Check sheet for the modelled part. Datum: model origin and axes. Units: mm. A direction names the side the tool comes from. Coordinates: 2 decimals unless noted, no trailing zeros. Write each loop counter-clockwise with the first axis right and the second up, starting at its lowest first coordinate (ties: lowest second). Pieces come first, ordered by that corner, then holes. Notation, with made-up numbers: (18, 85) - (22, 85) arc R21 ccw to (22, 97) - close; hole circle Ø3 at (-33.5, 39). An arc over 180 degrees is marked (long way). Answer as CSV lines item,"result". Start each with the question number.
from build123d import *
from build123d.topology import SkipClean

# Parameters (mm, degrees)
SKETCH1_R           = 21
SKETCH1_R_2         = 2.2
BOSS_EXTRUDE1_DEPTH = 7
SKETCH3_R           = 11.25
SKETCH3_R_2         = 2
BOSS_EXTRUDE2_DEPTH = 14
CUT_EXTRUDE1_START  = -1.5
SKETCH4_R           = 11.25
SKETCH4_R_2         = 9.9
CUT_EXTRUDE1_DEPTH  = 1.5
SKETCH5_R           = 2.2
CUT_EXTRUDE2_DEPTH  = 133.951156445
CUT_EXTRUDE3_DEPTH  = 6.5
CUT_EXTRUDE4_START  = -10
SKETCH7_R           = 2
CUT_EXTRUDE4_DEPTH  = 10
SKETCH8_R           = 2.2
CUT_EXTRUDE5_DEPTH  = 133.951156445
SKETCH9_R           = 4.15
CUT_EXTRUDE6_DEPTH  = 3
BOSS_EXTRUDE3_START = 17.5
SKETCH10_R          = 21
SKETCH10_R_2        = 2.2
BOSS_EXTRUDE3_DEPTH = 17.5
CUT_EXTRUDE7_DEPTH  = 17.5


with BuildPart() as part:
    # Sketch1 → Boss-Extrude1 (new body)
    with BuildSketch(Plane(origin=(0, 0, 0), x_dir=(1, 0, 0), z_dir=(0, 1, 0))):
        with BuildLine():
            Line((-112.6, -35.6), (-112.6, 35.6))
            Line((-112.6, 35.6), (-20.090163155, 64.440944627))
            ThreePointArc((-20.090163155, 64.440944627), (67.5, 0), (-20.090163155, -64.440944627))
            Line((-20.090163155, -64.440944627), (-112.6, -35.6))
        make_face()
        with Locations(Location((-77, 0, 0), (0, 0, 270))):
            Circle(SKETCH1_R, mode=Mode.SUBTRACT)
        with Locations(Location((-100.6, 23.6, 0), (0, 0, 270))):
            Circle(SKETCH1_R_2, mode=Mode.SUBTRACT)
        with Locations(Location((-100.6, -23.6, 0), (0, 0, 270))):
            Circle(SKETCH1_R_2, mode=Mode.SUBTRACT)
        with Locations(Location((-53.4, -23.6, 0), (0, 0, 270))):
            Circle(SKETCH1_R_2, mode=Mode.SUBTRACT)
        with Locations(Location((-53.4, 23.6, 0), (0, 0, 270))):
            Circle(SKETCH1_R_2, mode=Mode.SUBTRACT)
    extrude(amount=BOSS_EXTRUDE1_DEPTH)

    # Sketch3 → Boss-Extrude2 (add)
    with BuildSketch(Plane.XZ):
        with Locations(Location((0, 0, 0), (0, 0, 90))):
            Circle(SKETCH3_R)
        with Locations(Location((0, 0, 0), (0, 0, 270))):
            Circle(SKETCH3_R_2, mode=Mode.SUBTRACT)
    extrude(amount=BOSS_EXTRUDE2_DEPTH)

    # Sketch4 → Cut-Extrude1 (cut)
    with BuildSketch(Plane.XZ.offset(14).offset(CUT_EXTRUDE1_START)):
        with Locations(Location((0, 0, 0), (0, 0, 90))):
            Circle(SKETCH4_R)
        with Locations(Location((0, 0, 0), (0, 0, 270))):
            Circle(SKETCH4_R_2, mode=Mode.SUBTRACT)
    extrude(amount=CUT_EXTRUDE1_DEPTH, mode=Mode.SUBTRACT)

    # Sketch5 → Cut-Extrude2 (cut, through all)
    with BuildSketch(Plane.XZ.offset(14)):
        with Locations(Location((-7.6, 0, 0), (0, 0, 270))):
            Circle(SKETCH5_R)
        with Locations(Location((3.8, 6.581793069, 0), (0, 0, 270))):
            Circle(SKETCH5_R)
        with Locations(Location((3.8, -6.581793069, 0), (0, 0, 270))):
            Circle(SKETCH5_R)
    extrude(amount=-CUT_EXTRUDE2_DEPTH, mode=Mode.SUBTRACT)

    # Sketch6 → Cut-Extrude3 (cut)
    with BuildSketch(Plane(origin=(0, 7, 0), x_dir=(1, 0, 0), z_dir=(0, 1, 0))):
        Polygon((3.8, 2.33826859), (7.475, 4.460030829), (7.475, 8.703555308), (3.8, 10.825317547), (0.125, 8.703555308), (0.125, 4.460030829), align=None)
        Polygon((-7.6, -4.243524479), (-3.925, -2.121762239), (-3.925, 2.121762239), (-7.6, 4.243524479), (-11.275, 2.121762239), (-11.275, -2.121762239), align=None)
        Polygon((0.125, -4.460030829), (0.125, -8.703555308), (3.8, -10.825317547), (7.475, -8.703555308), (7.475, -4.460030829), (3.8, -2.33826859), align=None)
    extrude(amount=-CUT_EXTRUDE3_DEPTH, mode=Mode.SUBTRACT)

    # Sketch7 → Cut-Extrude4 (cut)
    with BuildSketch(Plane.XZ.offset(CUT_EXTRUDE4_START)):
        with Locations(Location((0, 0, 0), (0, 0, 90))):
            Circle(SKETCH7_R)
    extrude(amount=CUT_EXTRUDE4_DEPTH, mode=Mode.SUBTRACT)

    # Sketch8 → Cut-Extrude5 (cut, through all)
    with BuildSketch(Plane(origin=(0, 7, 0), x_dir=(1, 0, 0), z_dir=(0, 1, 0))):
        with Locations(Location((-28, 0, 0), (0, 0, 270))):
            Circle(SKETCH8_R)
        with Locations(Location((28, 0, 0), (0, 0, 270))):
            Circle(SKETCH8_R)
        with Locations(Location((28, 28, 0), (0, 0, 270))):
            Circle(SKETCH8_R)
        with Locations(Location((-28, 28, 0), (0, 0, 270))):
            Circle(SKETCH8_R)
        with Locations(Location((-28, -28, 0), (0, 0, 270))):
            Circle(SKETCH8_R)
        with Locations(Location((28, -28, 0), (0, 0, 270))):
            Circle(SKETCH8_R)
    extrude(amount=-CUT_EXTRUDE5_DEPTH, mode=Mode.SUBTRACT)

    # Sketch9 → Cut-Extrude6 (cut)
    with BuildSketch(Plane.XZ):
        with Locations(Location((-28, 28, 0), (0, 0, 270))):
            Circle(SKETCH9_R)
        with Locations(Location((28, 28, 0), (0, 0, 270))):
            Circle(SKETCH9_R)
        with Locations(Location((-28, 0, 0), (0, 0, 270))):
            Circle(SKETCH9_R)
        with Locations(Location((28, 0, 0), (0, 0, 270))):
            Circle(SKETCH9_R)
        with Locations(Location((-28, -28, 0), (0, 0, 270))):
            Circle(SKETCH9_R)
        with Locations(Location((28, -28, 0), (0, 0, 270))):
            Circle(SKETCH9_R)
    extrude(amount=-CUT_EXTRUDE6_DEPTH, mode=Mode.SUBTRACT)

    # Sketch10 → Boss-Extrude3 (add)
    with SkipClean():  # the faces are left unmerged after this step: merging them gives an invalid solid
        with BuildSketch(Plane.XZ.offset(BOSS_EXTRUDE3_START)):
            with BuildLine():
                Line((-20.090163155, -64.440944627), (-112.6, -35.6))
                Line((-112.6, -35.6), (-112.6, 35.6))
                Line((-112.6, 35.6), (-20.090163155, 64.440944627))
                add(Edge.make_bspline(
                    [(-20.090163155, 64.440944627), (-39.318301135, 35.015813189), (-40.987873114, 0)],
                    knots=[0, 0, 0, 1, 1, 1], degree=2))
                add(Edge.make_bspline(
                    [(-20.090163155, -64.440944627), (-39.318301135, -35.015813189), (-40.987873114, 0)],
                    knots=[0, 0, 0, 1, 1, 1], degree=2))
            make_face()
            with Locations(Location((-77, 0, 0), (0, 0, 270))):
                Circle(SKETCH10_R, mode=Mode.SUBTRACT)
            with Locations(Location((-100.6, 23.6, 0), (0, 0, 270))):
                Circle(SKETCH10_R_2, mode=Mode.SUBTRACT)
            with Locations(Location((-53.4, 23.6, 0), (0, 0, 270))):
                Circle(SKETCH10_R_2, mode=Mode.SUBTRACT)
            with Locations(Location((-53.4, -23.6, 0), (0, 0, 270))):
                Circle(SKETCH10_R_2, mode=Mode.SUBTRACT)
            with Locations(Location((-100.6, -23.6, 0), (0, 0, 270))):
                Circle(SKETCH10_R_2, mode=Mode.SUBTRACT)
        extrude(amount=-BOSS_EXTRUDE3_DEPTH)

    # Sketch11 → Cut-Extrude7 (cut)
    with BuildSketch(Plane(origin=(0, 7, 0), x_dir=(1, 0, 0), z_dir=(0, 1, 0))):
        with BuildLine():
            Line((-25.949987435, 68.270103726), (-139.321617663, 44.018727608))
            Line((-139.321617663, 44.018727608), (-144.313851883, -55.417541664))
            Line((-144.313851883, -55.417541664), (-25.949987435, -68.270103726))
            add(Edge.make_bspline(
                [(-47.995441412, -1e-09), (-47.925769838, -1.535411027), (-47.737002645, -4.611648854), (-47.165699577, -10.689341017), (-46.085583629, -18.188567618), (-44.203243401, -27.011172833), (-41.734657134, -35.6544225), (-38.681165485, -44.111018236), (-35.046062429, -52.374277572), (-31.533581002, -59.097437671), (-28.439841721, -64.370244449), (-26.792175769, -66.981289258), (-25.949987435, -68.270103726)],
                knots=[0.498938173, 0.498938173, 0.498938173, 0.498938173, 0.499072926, 0.49920768, 0.499477188, 0.499746696, 0.500016204, 0.500285712, 0.50055522, 0.500824727, 0.500959481, 0.501094235, 0.501094235, 0.501094235, 0.501094235], degree=3))
            add(Edge.make_bspline(
                [(-25.949987435, 68.270103726), (-26.792175769, 66.981289258), (-28.439841721, 64.370244449), (-31.533581002, 59.097437671), (-35.046062429, 52.374277572), (-38.681165485, 44.111018235), (-41.734657134, 35.654422499), (-44.203243402, 27.011172832), (-46.085583629, 18.188567617), (-47.165699577, 10.689341015), (-47.737002645, 4.611648852), (-47.925769838, 1.535411025), (-47.995441412, -1e-09)],
                knots=[0.498905765, 0.498905765, 0.498905765, 0.498905765, 0.499040519, 0.499175273, 0.49944478, 0.499714288, 0.499983796, 0.500253304, 0.500522812, 0.50079232, 0.500927074, 0.501061827, 0.501061827, 0.501061827, 0.501061827], degree=3))
        make_face()
    extrude(amount=-CUT_EXTRUDE7_DEPTH, mode=Mode.SUBTRACT)


solid = part.part
(1) Tool access check on faces 1 (the face through (32.115, 1.479, 0.54)), 2 (the face through (-2.3, -14, -0.1)), 3 (the face through (5.4, 0.5, 8.4)). Record the directions out of +Z, -Z, +X, -X, +Y, -Y that give a thin tool (end or side, any length) a straight path to the whole face; none if there is none.
(2) Cross-section at B-B on x = 28. Record the boundary of the cut face in (y, z), plus the area to 3 significant figures.
(3) Go/stop test with flat-tipped pins: P1, Ø1.3, axis at y = 4.5, z = -6.5, coming from the -X side; P2, Ø1, axis at x = 9, y = -13.5, coming from the -Z side; P3, Ø1.5, axis at x = 20, y = 0, coming from the -Z side. Record where each tip stops, or that it passes through.
(4) Material ranges on probe 1 along X at (y, z) = (0.8, -28); probe 2 along X at (y, z) = (-15, 0.5); probe 3 along Y at (x, z) = (-3.5, -12.5), recorded low to high. Write a range as from..to.
(5) Cross-section at A-A on x = -79.5. Record the boundary of the cut face in (y, z).
(6) Cross-section at D-D on x = -53.4. Record the boundary of the cut face in (y, z).
(7) Cross-section at C-C on y = -3.75. State how many separate pieces and enclosed holes the cut face has, plus the area to 3 significant figures.
Checked values:
1,face 1,"-Y"
1,face 2,"+Z, -Z, +X, -Y"
1,face 3,"+Y"
2,outline,"(0, -61.42) - (7, -61.42) - (7, -30.2) - (3, -30.2) - (3, -32.15) - (0, -32.15) - close; (0, -23.85) - (3, -23.85) - (3, -25.8) - (7, -25.8) - (7, -2.2) - (3, -2.2) - (3, -4.15) - (0, -4.15) - close; (0, 4.15) - (3, 4.15) - (3, 2.2) - (7, 2.2) - (7, 25.8) - (3, 25.8) - (3, 23.85) - (0, 23.85) - close; (0, 32.15) - (3, 32.15) - (3, 30.2) - (7, 30.2) - (7, 61.42) - (0, 61.42) - close"
2,area,"732 mm^2"
3,P1,"x = -47.61"
3,P2,"z = -5.08"
3,P3,"z = -64.7"
4,probe 1,"-43.85..-32.15, -23.85..23.85, 32.15..61.42"
4,probe 2,"-112.6..-97.99, -56.01..-40.96"
4,probe 3,"0..7"
5,outline,"(-17.5, -45.92) - (-10.5, -45.92) - (-10.5, -20.85) - (-17.5, -20.85) - close; (-17.5, 20.85) - (-10.5, 20.85) - (-10.5, 45.92) - (-17.5, 45.92) - close"
6,outline,"(-17.5, -54.06) - (-10.5, -54.06) - (-10.5, -25.8) - (-17.5, -25.8) - close; (-17.5, -21.4) - (-10.5, -21.4) - (-10.5, 21.4) - (-17.5, 21.4) - close; (-17.5, 25.8) - (-10.5, 25.8) - (-10.5, 54.06) - (-17.5, 54.06) - close"
7,separate pieces,"2"
7,enclosed holes,"4"
7,area,"1,270 mm^2"
